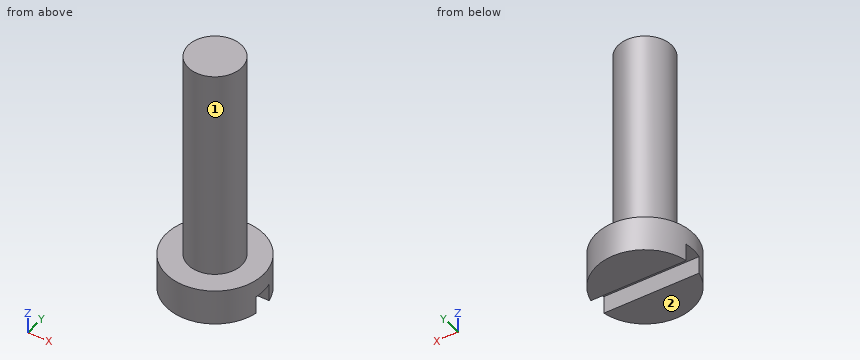
```python
from build123d import *

# Parameters (mm, degrees)
SKETCH1_R          = 2.725
EXTRUDE1_DEPTH     = 2
CUT_EXTRUDE1_DEPTH = 1
SKETCH3_R          = 1.5
EXTRUDE2_DEPTH     = 12


with BuildPart() as part:
    # Sketch1 → Extrude1 (new body)
    with BuildSketch(Plane.XY):
        Circle(SKETCH1_R)
    extrude(amount=EXTRUDE1_DEPTH)

    # Sketch2 → Cut-Extrude1 (cut)
    with BuildSketch(Plane(origin=(0, 0, 0), x_dir=(-1, 0, 0), z_dir=(0, 0, -1))):
        Polygon((3.449801909, 0), (3.449801909, 0.55), (-3.901269584, 0.55), (-3.901269584, -0.55), (3.449801909, -0.55), align=None)
    extrude(amount=-CUT_EXTRUDE1_DEPTH, mode=Mode.SUBTRACT)

    # Sketch3 → Extrude2 (add)
    with BuildSketch(Plane.XY.offset(2)):
        Circle(SKETCH3_R)
    extrude(amount=EXTRUDE2_DEPTH)


solid = part.part
```
The model under review builds one solid part; all positions refer to its coordinate system, in mm. Face numbers are marked on the shaded views. A direction names the side the tool comes from. Round coordinates to 2 decimals unless told otherwise and drop trailing zeros. Order: outer loops, then holes, each group sorted by start corner. A loop starts at its lowest first (then second) coordinate and runs counter-clockwise, first axis right, second up.
(1) Take a section at C-C, the plane z = 4.75. State the section outline as (x, y) points, plus the area to 3 significant figures.
Working result:
outline: circle Ø3 at (0, 0)
area: 7.07 mm2
(2) For P1, Ø1.5, axis at x = 2, z = 4.5, coming from the +Y side; P2, Ø1, axis at y = 0.5, z = 9, coming from the -X side; P3, Ø1.5, axis at x = 2, z = 7, coming from the -Y side, all flat-tipped, find the tip position at first contact; note any pin that passes through.
Working result:
P1: stops at y = 0.83
P2: stops at x = -1.5
P3: stops at y = -0.83
(3) Take a section at D-D, the plane x = -2.2. State the section outline as (y, z) points, plus the area to 3 significant figures.
Working result:
outline: (-1.61, 0) - (-0.55, 0) - (-0.55, 1) - (0.55, 1) - (0.55, 0) - (1.61, 0) - (1.61, 2) - (-1.61, 2) - close
area: 5.33 mm2
(4) Take a section at A-A, the plane x = 0. State the section outline as (y, z) points (3 decimals).
Working result:
outline: (-2.725, 0) - (-0.55, 0) - (-0.55, 1) - (0.55, 1) - (0.55, 0) - (2.725, 0) - (2.725, 2) - (1.5, 2) - (1.5, 14) - (-1.5, 14) - (-1.5, 2) - (-2.725, 2) - close
(5) Take a section at B-B, the plane y = 0. State the section outline as (x, z) points (3 decimals).
Working result:
outline: (-2.725, 1) - (2.725, 1) - (2.725, 2) - (1.5, 2) - (1.5, 14) - (-1.5, 14) - (-1.5, 2) - (-2.725, 2) - close
(6) Tool access review of the marked faces 1 and 2: name each direction out of +Z, -Z, +X, -X, +Y, -Y from which nothing blocks a thin tool from reaching the whole face with its end or side.
Working result:
face 1: +Z
face 2: -Z, +X, -X, +Y, -Y
(7) Wall thickness on L1, parallel to Z at x = -1.05, y = 1.85; L2, parallel to Z at x = -2.4, y = 0.4; L3, parallel to Y at x = 0.55, z = 1.5: over which ranges is each line inside the solid? List them lowest first.
Working result:
L1: z = 0 to 2
L2: z = 1 to 2
L3: y = -2.67 to 2.67
